The figure shows three views and two pictorial views of one solid part (mm, origin at its lowest corner). Answer the questions. Give positions to 0.01 mm unless a question says otherwise; leave off trailing zeros. Order: outer loops, then holes, each group sorted by start corner. A loop starts at its lowest first (then second) coordinate and runs counter-clockwise, first axis right, second up. Notation, with made-up numbers: (53, 0.5) -> (96, 0.5) arc R13 ccw to (96, 12.5) -> close; hole circle Ø2 at (40, 86). An arc over 180 degrees is marked (long way). Use one line per item in the form item = value.
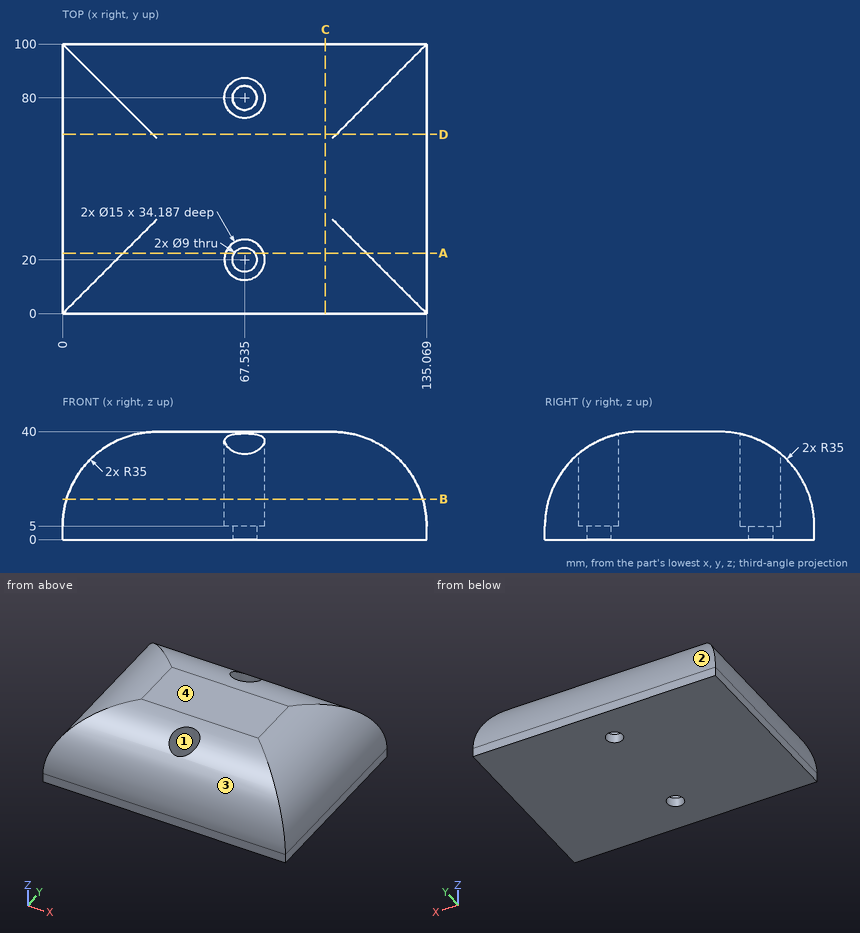
Item 1: The part is cut by section B-B on z = 15. Give the vertices of the cut face in (x, y) (1 decimal).
Checks:
outline = (1.5, 1.5) -> (133.6, 1.5) -> (133.6, 98.5) -> (1.5, 98.5) -> close; hole circle Ø15 at (67.5, 20); hole circle Ø15 at (67.5, 80)
Item 2: The part is cut by section C-C on x = 97.5. Give the vertices of the cut face in (y, z).
Checks:
outline = (0, 0) -> (100, 0) -> (100, 5) arc R35 ccw to (65, 40) -> (35, 40) arc R35 ccw to (0, 5) -> close
Item 3: Straight lines are drawn through the part: L1, parallel to X at y = 78, z = 8 (1 decimal); L2, parallel to Z at x = 119, y = 27; L3, parallel to Y at x = 21.5, z = 10. For each, find the intervals that lie inside material, in ascending order. Write a range as from..to.
Checks:
L1 = 0.1..60.3, 74.8..134.9
L2 = 0..34.44
L3 = 0.36..99.64
Item 4: The part is cut by section A-A on y = 22.5. Give the vertices of the cut face in (x, z) (1 decimal).
Checks:
outline = (0, 0) -> (63.8, 0) -> (63.8, 5) -> (60.5, 5) -> (60.5, 37.7) -> (22.5, 37.7) arc R35 ccw to (0, 5) -> close; (71.3, 0) -> (135.1, 0) -> (135.1, 5) arc R35 ccw to (112.6, 37.7) -> (74.6, 37.7) -> (74.6, 5) -> (71.3, 5) -> close
Item 5: The part is cut by section D-D on y = 66.5. Give the vertices of the cut face in (x, z), and give its area (4 significant figures).
Checks:
outline = (0, 0) -> (135.07, 0) -> (135.07, 5) arc R35 ccw to (101.57, 39.97) -> (33.5, 39.97) arc R35 ccw to (0, 5) -> close
area = 4,875 mm²
Item 6: Given pin 1 Ø10 at (y, z) = (38.5, 24) entering from -X; pin 2 Ø11.5 at (x, y) = (67.53, 20) entering from +Z; pin 3 Ø12 at (x, y) = (19.5, 82) entering from +Z; pin 4 Ø7 at (x, y) = (67.53, 80) entering from +Z, each flat-ended and moving along its own axis, determine where each tip first touches the part or whether it passes through.
Checks:
pin_1 = 2.92
pin_2 = 5
pin_3 = 37.85
pin_4 = through
Item 7: Determine the mould class of the marked faces 1, 2, 3 and 4 for opening direction Y: +Y half, -Y half, draft (parallel to the pull), parting line (faces both ways), or undercut.
Checks:
face_1 = undercut
face_2 = +Y half
face_3 = -Y half
face_4 = draft
